Could you check a few things on this model? Use its own coordinates, in mm. Face numbers are marked on the shaded views. Give positions to 0.01 mm unless a question says otherwise; leave off trailing zeros. Loops run counter-clockwise (first coordinate to the right, second up) from the corner with the lowest first, then second, coordinate; pieces in that order, holes last. Notation, with made-up numbers: (32, 42.25) -> (39, 42.25) arc R28 cw to (39, 64.25) -> close; hole circle Ø10 at (31, -9). An arc over 180 degrees is marked (long way). Put each result on its own line as item: value.
```python
from build123d import *

# Parameters (mm, degrees)
SKETCH1_R           = 35
SKETCH1_R_2         = 5
SKETCH1_R_3         = 2.5
BOSS_EXTRUDE1_DEPTH = 45
SKETCH2_R           = 16
CUT_EXTRUDE1_DEPTH  = 5
SKETCH5_R           = 13
CUT_EXTRUDE2_DEPTH  = 40
SKETCH6_R           = 13
BOSS_EXTRUDE2_DEPTH = 18


with BuildPart() as part:
    # Sketch1 → Boss-Extrude1 (new body)
    with BuildSketch(Plane(origin=(0, 0, 0), x_dir=(1, 0, 0), z_dir=(0, 1, 0))):
        with Locations(Location((0, 0, 0), (0, 0, 90))):
            Circle(SKETCH1_R)
        with Locations(Location((0, 0, 0), (0, 0, 90))):
            Circle(SKETCH1_R_2, mode=Mode.SUBTRACT)
        with Locations(Location((0, 22.5, 0), (0, 0, 90))):
            Circle(SKETCH1_R_3, mode=Mode.SUBTRACT)
        with Locations(Location((19.485571585, 11.25, 0), (0, 0, 90))):
            Circle(SKETCH1_R_3, mode=Mode.SUBTRACT)
        with Locations(Location((19.485571585, -11.25, 0), (0, 0, 90))):
            Circle(SKETCH1_R_3, mode=Mode.SUBTRACT)
        with Locations(Location((0, -22.5, 0), (0, 0, 90))):
            Circle(SKETCH1_R_3, mode=Mode.SUBTRACT)
        with Locations(Location((-19.485571585, -11.25, 0), (0, 0, 90))):
            Circle(SKETCH1_R_3, mode=Mode.SUBTRACT)
        with Locations(Location((-19.485571585, 11.25, 0), (0, 0, 90))):
            Circle(SKETCH1_R_3, mode=Mode.SUBTRACT)
    extrude(amount=BOSS_EXTRUDE1_DEPTH)

    # Sketch2 → Cut-Extrude1 (cut)
    with BuildSketch(Plane.XZ):
        with Locations(Location((0, 0, 0), (0, 0, 270))):
            Circle(SKETCH2_R)
    extrude(amount=-CUT_EXTRUDE1_DEPTH, mode=Mode.SUBTRACT)

    # Sketch5 → Cut-Extrude2 (cut)
    with BuildSketch(Plane(origin=(0, 45, 0), x_dir=(1, 0, 0), z_dir=(0, 1, 0))):
        with Locations(Location((0, 0, 0), (0, 0, 270))):
            Circle(SKETCH5_R)
    extrude(amount=-CUT_EXTRUDE2_DEPTH, mode=Mode.SUBTRACT)

    # Sketch6 → Boss-Extrude2 (add)
    with BuildSketch(Plane(origin=(0, 45, 0), x_dir=(1, 0, 0), z_dir=(0, 1, 0))):
        with Locations(Location((0, 0, 0), (0, 0, 270))):
            Circle(SKETCH6_R)
    extrude(amount=-BOSS_EXTRUDE2_DEPTH)


solid = part.part
```
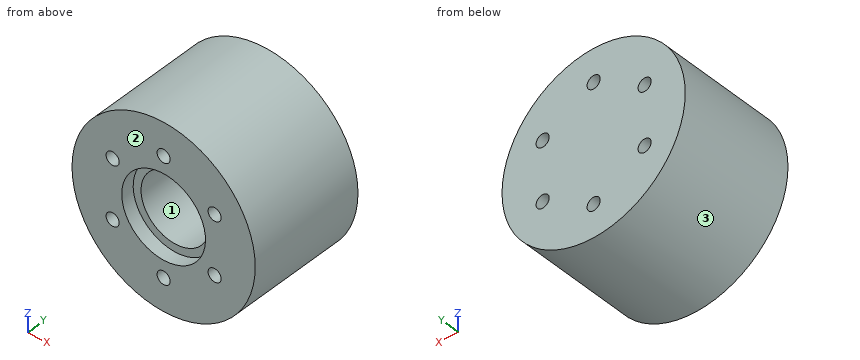
1. If we section it at D-D (y = 34.5): List the corners of the cut face in (x, z) for me, then the cut area to 3 significant figures.
Recorded:
outline: circle Ø70 at (0, 0); hole circle Ø5 at (-19.49, -11.25); hole circle Ø5 at (-19.49, 11.25); hole circle Ø5 at (0, -22.5); hole circle Ø5 at (0, 22.5); hole circle Ø5 at (19.49, -11.25); hole circle Ø5 at (19.49, 11.25)
area: 3,730 mm^2
2. I need wall thicknesses on line 1 (X direction, y = 1.5, z = 0); line 2 (Z direction, x = 1, y = 4.5); line 3 (Z direction, x = -17.5, y = 38). Which ranges of each line are inside material? Lowest first, please.
Recorded:
line 1: x = -35 to -16, 16 to 35
line 2: z = -34.99 to -24.79, -20.21 to -15.97, 15.97 to 20.21, 24.79 to 34.99
line 3: z = -30.31 to -12.77, -9.73 to 9.73, 12.77 to 30.31
3. Thinking about a two-plate mould opening in Z: for the marked faces 1, 2 and 3, which applies, pulls with the +Z half, pulls with the -Z half, needs draft (parallel to the pull), parting line crosses it, or undercut?
Recorded:
face 1: undercut
face 2: needs draft
face 3: parting line crosses it
4. If we section it at B-B (z = -11.25): List the corners of the cut face in (x, y) for me.
Recorded:
outline: (-33.14, 0) -> (-21.99, 0) -> (-21.99, 45) -> (-33.14, 45) -> close; (-16.99, 0) -> (-11.38, 0) -> (-11.38, 5) -> (-6.51, 5) -> (-6.51, 27) -> (6.51, 27) -> (6.51, 5) -> (11.38, 5) -> (11.38, 0) -> (16.99, 0) -> (16.99, 45) -> (-16.99, 45) -> close; (21.99, 0) -> (33.14, 0) -> (33.14, 45) -> (21.99, 45) -> close
5. If we section it at C-C (y = 6.5): List the corners of the cut face in (x, z) for me, then the cut area to 3 significant figures.
Recorded:
outline: circle Ø70 at (0, 0); hole circle Ø5 at (-19.49, -11.25); hole circle Ø5 at (-19.49, 11.25); hole circle Ø26 at (0, 0); hole circle Ø5 at (0, -22.5); hole circle Ø5 at (0, 22.5); hole circle Ø5 at (19.49, -11.25); hole circle Ø5 at (19.49, 11.25)
area: 3,200 mm^2
6. I'm going to push flat-ended pins straight in: pin 1 (1 mm diameter, centred on y = 9, z = 27, fed in from +X); pin 2 (1.5 mm diameter, centred on x = -16.5, y = 19.5, fed in from +Z); pin 3 (5 mm diameter, centred on x = -10.5, y = 19.5, fed in from -Z); pin 4 (4.5 mm diameter, centred on x = 19.49, z = -11.25, fed in from +Y). Where does each tip first touch, or does it pass through?
Recorded:
pin 1: stops at x = 22.86
pin 2: stops at z = 31.26
pin 3: stops at z = -34.07
pin 4: passes through
7. If we section it at A-A (x = 0): List the corners of the cut face in (y, z) for me.
Recorded:
outline: (0, -35) -> (45, -35) -> (45, -25) -> (0, -25) -> close; (0, -20) -> (45, -20) -> (45, 20) -> (0, 20) -> (0, 16) -> (5, 16) -> (5, 13) -> (27, 13) -> (27, -13) -> (5, -13) -> (5, -16) -> (0, -16) -> close; (0, 25) -> (45, 25) -> (45, 35) -> (0, 35) -> close
